```python
from build123d import *

# Parameters (mm, degrees)
EXTRUDE_1_DEPTH     = 10
SKETCH_2_R          = 3.25
CUT_EXTRUDE_1_DEPTH = 65.845971347
SKETCH_4_W          = 13
SKETCH_4_H          = 24.888888889
CUT_EXTRUDE_2_DEPTH = 7.5


with BuildPart() as part:
    # 草图1 → 凸台-拉伸1 (new, symmetric)
    with BuildSketch(Plane(origin=(0, 0, 0), x_dir=(1, 0, 0), z_dir=(0, 1, 0))):
        Polygon((-53, -18), (-35, -18), (-35, 12), (35, 12), (35, -18), (53, -18), (53, -4), (35, 18), (-35, 18), (-53, -4), align=None)
    extrude(amount=EXTRUDE_1_DEPTH, both=True)

    # 草图2 → 切除-拉伸1 (cut, through all)
    with BuildSketch(Plane.XY.offset(18)):
        with Locations((-45, 0)):
            Circle(SKETCH_2_R)
        with Locations((45, 0)):
            Circle(SKETCH_2_R)
    extrude(amount=-CUT_EXTRUDE_1_DEPTH, mode=Mode.SUBTRACT)

    # 草图4 → 切除-拉伸2 (cut, symmetric)
    with BuildSketch(Plane(origin=(0, 0, 0), x_dir=(1, 0, 0), z_dir=(0, 1, 0))):
        with Locations((46.5, -0.555555555)):
            Rectangle(SKETCH_4_W, SKETCH_4_H)
        with Locations((-46.5, -0.555555555)):
            Rectangle(SKETCH_4_W, SKETCH_4_H)
    extrude(amount=CUT_EXTRUDE_2_DEPTH, both=True, mode=Mode.SUBTRACT)


solid = part.part
```
Part model, mm, in its own coordinate system. A direction names the side the tool comes from. Round coordinates to 2 decimals unless told otherwise and drop trailing zeros. Write each loop counter-clockwise with the first axis right and the second up, starting at its lowest first coordinate (ties: lowest second). Pieces come first, ordered by that corner, then holes. Notation, with made-up numbers: M -18,6.5 L 25,6.5 A14 cw 25,25.5 Z; hole C 85.5,48.25 d8. An arc over 180 degrees is marked long. One line per question, with ' | ' between items.
(1) Pin check, flat tips, straight feed: pin 1 (6 mm diameter, centred on x = 16.5, y = -3.5, fed in from +Z); pin 2 (7.5 mm diameter, centred on y = -1.5, z = -0.5, fed in from +X); pin 3 (8 mm diameter, centred on x = -23.5, z = -6.5, fed in from -Y); pin 4 (6 mm diameter, centred on y = -0.5, z = -1.5, fed in from -X). Stop position of each tip, or through.
Answer key:
pin 1: stops at z = -12 | pin 2: stops at x = 40 | pin 3: passes through | pin 4: stops at x = -40
(2) Saw through at A-A on z = 5. Write the cut outline in (x, y), then the cut area to 3 significant figures.
Answer key:
outline: M -53,-10 L -35,-10 L -35,10 L -53,10 L -53,7.5 L -40,7.5 L -40,-7.5 L -53,-7.5 Z; M 35,-10 L 53,-10 L 53,-7.5 L 40,-7.5 L 40,7.5 L 53,7.5 L 53,10 L 35,10 Z | area: 330 mm^2
(3) 3-axis set-ups, long thin cutter, end or side, ignore diameter. For faces 1 (the face through (0, 0, -12)), 2 (the face through (-45, 7.5, 3)), 3 (the face through (45, -7.5, 3)): which of +Z, -Z, +X, -X, +Y, -Y reach the whole face in a straight line?
Answer key:
face 1: +Z, +Y, -Y | face 2: -Z, -X | face 3: -Z, +X
(4) Saw through at D-D on y = 6. Write the cut outline in (x, z), then the cut area to 3 significant figures.
Answer key:
outline: M -53,13 L -40,13 L -40,-11.89 L -35,-18 L 35,-18 L 40,-11.89 L 40,13 L 53,13 L 53,18 L 35,18 L 35,-12 L -35,-12 L -35,18 L -53,18 Z | area: 879 mm^2
(5) Probe line 1 along X through (y, z) = (0.5, 10.5); line 2 along Y through (x, z) = (43.5, -3.5); line 3 along Y through (x, z) = (-45, 16.15). List the from-to ranges inside material, lowest first.
Answer key:
line 1: x = -40 to -35, 35 to 40 | line 2: y = -10 to -7.5, 7.5 to 10 | line 3: y = -10 to -3.25, 3.25 to 10
(6) Saw through at B-B on x = 45. Write the cut outline in (y, z), then the cut area to 3 significant figures.
Answer key:
outline: M -10,-5.78 L -7.5,-5.78 L -7.5,13 L -3.25,13 L -3.25,18 L -10,18 Z; M 3.25,13 L 7.5,13 L 7.5,-5.78 L 10,-5.78 L 10,18 L 3.25,18 Z | area: 161 mm^2
(7) Saw through at C-C on y = 0. Write the cut outline in (x, z).
Answer key:
outline: M -53,13 L -48.25,13 L -48.25,18 L -53,18 Z; M -41.75,13 L -40,13 L -40,-11.89 L -35,-18 L 35,-18 L 40,-11.89 L 40,13 L 41.75,13 L 41.75,18 L 35,18 L 35,-12 L -35,-12 L -35,18 L -41.75,18 Z; M 48.25,13 L 53,13 L 53,18 L 48.25,18 Z
(8) Two-plate mould, pull along Y, no slides. Class faces 4 (the face through (45, 7.5, 3)), 5 (the face through (35, 0, 3)), 6 (the face through (-45, -7.5, 3)), 7 (the face through (-12.5, -10, -12.3)): released by +Y, released by -Y, zero draft, split by the parting line, or undercut.
Answer key:
face 4: undercut | face 5: zero draft | face 6: undercut | face 7: released by -Y
